The model under review builds one solid part; all positions refer to its coordinate system, in mm. Face numbers are marked on the shaded views. A direction names the side the tool comes from. Coordinates: 2 decimals unless noted, no trailing zeros. Order: outer loops, then holes, each group sorted by start corner. A loop starts at its lowest first (then second) coordinate and runs counter-clockwise, first axis right, second up. Notation, with made-up numbers: (73, -8) -> (120, -8) arc R12 ccw to (120, 14) -> close; hole circle Ø11 at (-6.75, -3). An arc over 180 degrees is marked (long way). Use one line per item in the form item = value.
Autodesk Inventor part; units mm, degrees
ref_plane "YZ Plane" through (0, 0, 0) normal (1, 0, 0) x (0, 1, 0)
ref_plane "XZ Plane" through (0, 0, 0) normal (0, 1, 0) x (-1, 0, 0)
ref_plane "XY Plane" through (0, 0, 0) normal (0, 0, 1) x (1, 0, 0)
sketch "スケッチ1" plane through (0, 0, 0) normal (1, 0, 0) x (0, 1, 0)
  circle A0 centre (0, 0) radius 17.5
  dimension "d0" = 35
extrude "押し出し1" add sketch "スケッチ1" along normal blind 3
sketch "スケッチ2" plane through (3, 0, 0) normal (1, 0, 0) x (0, 0, -1)
  circle A0 centre (0, 0) radius 13.5
  point P0 (13.5, 0)
  point P1 (6.75, 11.6913)
  point P2 (-6.75, 11.6913)
  point P3 (-13.5, 0)
  point P4 (-6.75, -11.6913)
  point P5 (6.75, -11.6913)
  dimension "d3" = 27
  dimension "d6" = 360
hole "穴1" at (3, 0, -13.5) at (3, 11.6913, -6.75) at (3, 11.6913, 6.75) at (3, 0, 13.5) at (3, -11.6913, 6.75) at (3, -11.6913, -6.75) direction (-1, 0, 0) diameter 3.2 end through all
sketch "スケッチ4" plane through (3, 0, 0) normal (1, 0, 0) x (0, 0, -1)
  circle A0 centre (0, 0) radius 25
  circle A1 centre (0, -25) radius 5
  circle A2 centre (0, 25) radius 5
  circle A3 centre (13.5, 0) radius 1.6
  circle A4 centre (-13.5, 0) radius 1.6
  line L0 (-1.8583, 31.7813) -> (-19.7652, 0.7657)
  line L1 (-19.9094, -0.516) -> (-0.3337, -34.4219)
  line L2 (1.1974, -32.9261) -> (19.8479, -0.6225)
  line L3 (2.1736, 31.2353) -> (21.8646, -2.8706)
  circle A5 centre (0, 0) radius 17.5
  point P0 (-4.3301, 27.5)
  point P1 (-15.1554, 8.75)
  point P2 (-15.1554, -8.75)
  point P3 (-4.3301, -27.5)
  point P4 (4.3301, -27.5)
  point P5 (15.1554, -8.75)
  point P6 (15.1554, 8.75)
  point P7 (4.3301, 27.5)
  dimension "d22" = 50
  dimension "d23" = 10
  dimension "d24" = 10
  dimension "d25" = 13.5
  dimension "d26" = 13.5
extrude "押し出し2" add sketch "スケッチ4" along normal blind 3 contours L3 A5 L0 A0 A2 | A0 A2 L3 | L2 A1 A0 | A0 A1 L1 A5 L2 | A2 A0 | A0 A2 | A5 | A1 A0 | A0 A1 | A0 L0 A2 | A1 L1 A0 | A3 | A4
sketch "スケッチ6" plane through (6, 0, 0) normal (1, 0, 0) x (0, 0, -1)
  arc A0 (4.3301, 27.5) -> (-4.3301, 27.5) centre (0, 25) ccw
  circle A1 centre (0, 25) radius 5
  arc A2 (-4.3301, -27.5) -> (4.3301, -27.5) centre (0, -25) ccw
  circle A3 centre (0, -25) radius 5
  point P0 (0, 0)
  point P1 (-4.3301, 27.5)
  point P2 (4.3301, 27.5)
  dimension "d29" = 10
  dimension "d30" = 10
extrude "押し出し3" add sketch "スケッチ6" along normal blind 3
sketch "スケッチ7" plane through (0, 0, 0) normal (-1, 0, 0) x (0, 0, 1)
  circle A0 centre (6.75, 11.6913) radius 1.6
  circle A1 centre (13.5, 0) radius 1.6
  circle A2 centre (6.75, -11.6913) radius 1.6
  circle A3 centre (-6.75, -11.6913) radius 1.6
  circle A4 centre (-13.5, 0) radius 1.6
  circle A5 centre (-6.75, 11.6913) radius 1.6
  arc A6 (4.3301, 27.5) -> (-4.3301, 27.5) centre (0, 25) ccw
  arc A7 (-4.3301, -27.5) -> (4.3301, -27.5) centre (0, -25) ccw
  point P0 (0, 0)
hole "穴2" at (0, 11.6913, 6.75) at (0, 0, 13.5) at (0, -11.6913, 6.75) at (0, -11.6913, -6.75) at (0, 0, -13.5) at (0, 11.6913, -6.75) at (0, 25, 0) at (0, -25, 0) direction (1, 0, 0) diameter 3.2 end through all
sketch "スケッチ9" plane through (0, 0, 0) normal (-1, 0, 0) x (0, 0, 1)
  circle A0 centre (0, 25) radius 1.6
  circle A1 centre (0, 25) radius 3.5
  circle A2 centre (0, -25) radius 1.6
  circle A3 centre (0, -25) radius 3.5
  point P0 (0, 0)
  point P1 (0.5822, 17.4903)
  point P2 (-0.5822, 17.4903)
  point P3 (-0.5822, -17.4903)
  point P4 (0.5822, -17.4903)
  dimension "d40" = 7
  dimension "d41" = 7
extrude "押し出し4" cut sketch "スケッチ9" against normal blind 7 contours A0 | A1 | A2 | A3
properties part number "endeff_3dp2" material "ABS プラスチック"
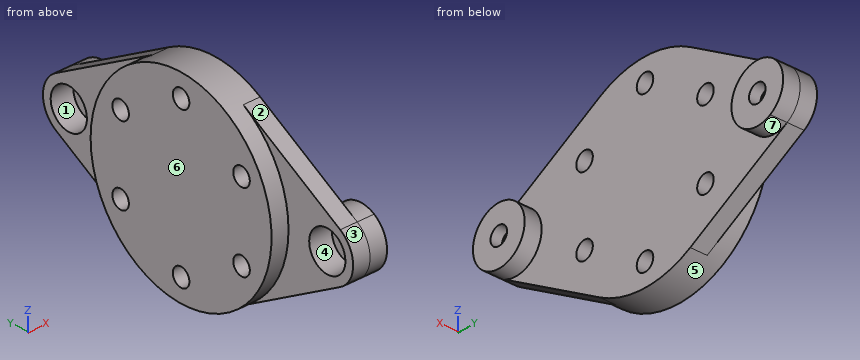
Item 1: We need section D-D (y = -25). Write out the cut boundary in (x, z).
Results found:
outline = (3, -5.77) -> (6, -5.77) -> (6, -5) -> (9, -5) -> (9, -1.6) -> (7, -1.6) -> (7, -3.5) -> (3, -3.5) -> close; (3, 3.5) -> (7, 3.5) -> (7, 1.6) -> (9, 1.6) -> (9, 5) -> (6, 5) -> (6, 5.77) -> (3, 5.77) -> close
Item 2: We need section C-C (x = 4). State how many separate pieces and enclosed holes the cut face has, plus the area to 3 significant figures.
Results found:
separate_pieces = 1
enclosed_holes = 8
area = 1,220 mm²
Item 3: Clearance check with flat-ended pins moving along their axes: pin 1 (2 mm diameter, centred on x = 3, y = 9, fed in from -Z); pin 2 (1.5 mm diameter, centred on x = 1, z = -9.5, fed in from +Y); pin 3 (3.5 mm diameter, centred on y = 11.69, z = 6.75, fed in from +X). State where each tip first meets the part, or that it passes through.
Results found:
pin_1 = -15.56
pin_2 = 15.16
pin_3 = 6
Item 4: We need section A-A (z = 0). Write out the cut boundary in (x, y).
Results found:
outline = (0, -17.5) -> (3, -17.5) -> (3, -21.5) -> (7, -21.5) -> (7, -23.4) -> (9, -23.4) -> (9, -20) -> (6, -20) -> (6, 20) -> (9, 20) -> (9, 23.4) -> (7, 23.4) -> (7, 21.5) -> (3, 21.5) -> (3, 17.5) -> (0, 17.5) -> close; (3, -30) -> (9, -30) -> (9, -26.6) -> (7, -26.6) -> (7, -28.5) -> (3, -28.5) -> close; (3, 28.5) -> (7, 28.5) -> (7, 26.6) -> (9, 26.6) -> (9, 30) -> (3, 30) -> close
Item 5: Tool access review of the marked faces 5, 6 and 7: name each direction out of +Z, -Z, +X, -X, +Y, -Y from which nothing blocks a thin tool from reaching the whole face with its end or side.
Results found:
face_5 = -X
face_6 = +Z, -Z, -X, +Y, -Y
face_7 = +X
Item 6: To check wall thickness, follow L1, parallel to Y at x = 4.55, z = 0; L2, parallel to Z at x = 8.5, y = 25; L3, parallel to Y at x = 4, z = 3. State the ranges of each line that lie inside material, in increasing order. Write a range as from..to.
Results found:
L1 = -30..-28.5, -21.5..21.5, 28.5..30
L2 = -5..-1.6, 1.6..5
L3 = -29..-26.8, -23.2..23.2, 26.8..29
Item 7: Draft analysis for pull direction Z (two halves, no side actions). For the marked faces 1, 2, 3 and 4, state which applies: released by +Z, released by -Z, zero draft, split by the parting line, or undercut.
Results found:
face_1 = undercut
face_2 = released by +Z
face_3 = split by the parting line
face_4 = undercut
Item 8: We need section B-B (y = 0). Write out the cut boundary in (x, z), plus the area to 3 significant figures.
Results found:
outline = (0, -17.5) -> (6, -17.5) -> (6, -15.1) -> (0, -15.1) -> close; (0, -11.9) -> (6, -11.9) -> (6, 11.9) -> (0, 11.9) -> close; (0, 15.1) -> (6, 15.1) -> (6, 17.5) -> (0, 17.5) -> close
area = 172 mm²
